from build123d import *

# Parameters (mm, degrees)
BOSS_EXTRUDE2_DEPTH = 5
BOSS_EXTRUDE3_DEPTH = 2
SKETCH4_W           = 3.2
SKETCH4_H           = 3.2
CUT_EXTRUDE1_DEPTH  = 2.5
SKETCH5_W           = 3.2
SKETCH5_H           = 3.2
CUT_EXTRUDE2_DEPTH  = 2.5
CUT_EXTRUDE4_REACH  = 34.123
CUT_EXTRUDE5_REACH  = 34.123
SKETCH8_W           = 2.5
SKETCH8_H           = 7
BOSS_EXTRUDE4_DEPTH = 5.96
SKETCH10_W          = 7
SKETCH10_H          = 2.49
BOSS_EXTRUDE5_DEPTH = 3
SKETCH11_W          = 7
SKETCH11_H          = 2.49
BOSS_EXTRUDE6_DEPTH = 5
SKETCH12_W          = 17
SKETCH12_H          = 2.5
BOSS_EXTRUDE7_DEPTH = 10
CUT_EXTRUDE7_REACH  = 41.734
SKETCH14_W          = 13
SKETCH14_H          = 8.75
SKETCH16_W          = 17
SKETCH16_H          = 1.25
BOSS_EXTRUDE8_DEPTH = 9.5
CUT_EXTRUDE8_REACH  = 34.394
SKETCH17_R          = 3.51
FILLET7_R           = 2
FILLET8_R           = 5
FILLET9_R           = 5
CHAMFER1_SIZE       = 2
CHAMFER2_SIZE       = 2
FILLET11_R          = 2
FILLET12_R          = 2
FILLET13_R          = 2
FILLET14_R          = 2
FILLET16_R          = 2


with BuildPart() as part:
    # Sketch2 → Boss-Extrude2 (new body)
    with BuildSketch(Plane.XY):
        Polygon((15.905331571, 19.450007488), (-15.905331571, 19.450007488), (-20.223253942, 15.132085117), (-21.991020895, 16.89985207), (-16.54629868, 22.344574285), (16.54629868, 22.344574285), (21.991020895, 16.89985207), (20.223253942, 15.132085117), align=None)
    extrude(amount=BOSS_EXTRUDE2_DEPTH)

    # Sketch2_2 → Boss-Extrude3 (add)
    with BuildSketch(Plane.XY):
        Polygon((15.905331571, 19.450007488), (-15.905331571, 19.450007488), (-20.223253942, 15.132085117), (-21.991020895, 16.89985207), (-16.54629868, 22.344574285), (16.54629868, 22.344574285), (21.991020895, 16.89985207), (20.223253942, 15.132085117), align=None)
    extrude(amount=-BOSS_EXTRUDE3_DEPTH)

    # Sketch4 → Cut-Extrude1 (cut)
    with BuildSketch(Plane(origin=(19.445436483, 19.445436483, 0), x_dir=(0.7071067811865479, -0.7071067811865471, 0), z_dir=(0.7071067811865471, 0.7071067811865479, 0))):
        with Locations((0, -1.5)):
            Rectangle(SKETCH4_W, SKETCH4_H)
    extrude(amount=-CUT_EXTRUDE1_DEPTH, mode=Mode.SUBTRACT)

    # Sketch5 → Cut-Extrude2 (cut)
    with BuildSketch(Plane(origin=(-19.445436483, 19.445436483, 0), x_dir=(0, 0, 1), z_dir=(-0.7071067811865477, 0.7071067811865475, 0))):
        with Locations((1.5, 0)):
            Rectangle(SKETCH5_W, SKETCH5_H)
    extrude(amount=-CUT_EXTRUDE2_DEPTH, mode=Mode.SUBTRACT)

    # Sketch6 → Cut-Extrude4 (cut, up to next)
    with BuildSketch(Plane.XY.offset(5), mode=Mode.PRIVATE) as cut_extrude4_sk1:
        Polygon((-20.011121908, 18.879751058), (-18.950461736, 19.940411229), (-17.182694783, 18.172644276), (-18.243354955, 17.111984105), align=None)
    cut_extrude4_tool1 = extrude(cut_extrude4_sk1.sketch, amount=-CUT_EXTRUDE4_REACH, mode=Mode.PRIVATE) & part.part
    add(cut_extrude4_tool1.solids().sort_by_distance((-18.596908, 18.526198, 5))[0], mode=Mode.SUBTRACT)

    # Sketch7 → Cut-Extrude5 (cut, up to next)
    with BuildSketch(Plane.XY.offset(5), mode=Mode.PRIVATE) as cut_extrude5_sk1:
        Polygon((17.182694783, 18.172644276), (18.950461736, 19.940411229), (20.011121908, 18.879751058), (18.243354955, 17.111984105), align=None)
    cut_extrude5_tool1 = extrude(cut_extrude5_sk1.sketch, amount=-CUT_EXTRUDE5_REACH, mode=Mode.PRIVATE) & part.part
    add(cut_extrude5_tool1.solids().sort_by_distance((18.596908, 18.526198, 5))[0], mode=Mode.SUBTRACT)

    # Sketch8 → Boss-Extrude4 (add)
    with BuildSketch(Plane(origin=(0, 19.450007488, 0), x_dir=(-1, 0, 0), z_dir=(0, -1, 0))):
        with Locations((11.1, -1.5)):
            Rectangle(SKETCH8_W, SKETCH8_H)
        with Locations((-11.1, -1.5)):
            Rectangle(SKETCH8_W, SKETCH8_H)
    extrude(amount=BOSS_EXTRUDE4_DEPTH)

    # Sketch10 → Boss-Extrude5 (add)
    with BuildSketch(Plane.ZY.offset(-9.85)):
        with Locations((1.5, 14.735007488)):
            Rectangle(SKETCH10_W, SKETCH10_H)
    extrude(amount=BOSS_EXTRUDE5_DEPTH)

    # Sketch11 → Boss-Extrude6 (add)
    with BuildSketch(Plane(origin=(-9.85, 0, 0), x_dir=(0, 0, -1), z_dir=(1, 0, 0))):
        with Locations((-1.5, 14.735007488)):
            Rectangle(SKETCH11_W, SKETCH11_H)
    extrude(amount=BOSS_EXTRUDE6_DEPTH)

    # Sketch12 → Boss-Extrude7 (add)
    with BuildSketch(Plane(origin=(0, 22.344574285, 0), x_dir=(1, 0, 0), z_dir=(0, 1, 0))):
        with Locations((0, -3.75)):
            Rectangle(SKETCH12_W, SKETCH12_H)
    extrude(amount=BOSS_EXTRUDE7_DEPTH)

    # Sketch14 → Cut-Extrude7 (cut, up to next)
    with BuildSketch(Plane.XY.offset(5), mode=Mode.PRIVATE) as cut_extrude7_sk1:
        with Locations((0, 26.719574285)):
            Rectangle(SKETCH14_W, SKETCH14_H)
    cut_extrude7_tool1 = extrude(cut_extrude7_sk1.sketch, amount=-CUT_EXTRUDE7_REACH, mode=Mode.PRIVATE) & part.part
    add(cut_extrude7_tool1.solids().sort_by_distance((0, 26.719574, 5))[0], mode=Mode.SUBTRACT)

    # Sketch16 → Boss-Extrude8 (add)
    with BuildSketch(Plane.XY.offset(5)):
        with Locations((0, 31.719574285)):
            Rectangle(SKETCH16_W, SKETCH16_H)
    extrude(amount=BOSS_EXTRUDE8_DEPTH)

    # Sketch17 → Cut-Extrude8 (cut, up to next)
    with BuildSketch(Plane(origin=(0, 32.344574285, 0), x_dir=(1, 0, 0), z_dir=(0, 1, 0)), mode=Mode.PRIVATE) as cut_extrude8_sk1:
        with Locations(Location((0, -9, 0), (0, 0, 270))):
            Circle(SKETCH17_R)
    cut_extrude8_tool1 = extrude(cut_extrude8_sk1.sketch, amount=-CUT_EXTRUDE8_REACH, mode=Mode.PRIVATE) & part.part
    add(cut_extrude8_tool1.solids().sort_by_distance((0, 32.344574, 9))[0], mode=Mode.SUBTRACT)

    # Fillet7
    fillet7_edges = [part.edges().sort_by_distance(p)[0] for p in [
        (7.5, 31.094574285, 5),
    ]]
    fillet(fillet7_edges, radius=FILLET7_R)

    # Fillet8
    fillet8_edges = [part.edges().sort_by_distance(p)[0] for p in [
        (8.5, 31.719574285, 14.5),
    ]]
    fillet(fillet8_edges, radius=FILLET8_R)

    # Fillet9
    fillet9_edges = [part.edges().sort_by_distance(p)[0] for p in [
        (-8.5, 31.719574285, 14.5),
    ]]
    fillet(fillet9_edges, radius=FILLET9_R)

    # Chamfer1
    chamfer1_edges = [part.edges().sort_by_distance(p)[0] for p in [
        (-12.35, 13.490007488, 1.5),
    ]]
    chamfer(chamfer1_edges, length=CHAMFER1_SIZE)

    # Chamfer2
    chamfer2_edges = [part.edges().sort_by_distance(p)[0] for p in [
        (12.35, 13.490007488, 1.5),
    ]]
    chamfer(chamfer2_edges, length=CHAMFER2_SIZE)

    # Fillet11
    fillet11_edges = [part.edges().sort_by_distance(p)[0] for p in [
        (-8.5, 22.344574285, 3.75),
    ]]
    fillet(fillet11_edges, radius=FILLET11_R)

    # Fillet12
    fillet12_edges = [part.edges().sort_by_distance(p)[0] for p in [
        (8.5, 22.344574285, 3.75),
    ]]
    fillet(fillet12_edges, radius=FILLET12_R)

    # Fillet13
    fillet13_edges = [part.edges().sort_by_distance(p)[0] for p in [
        (8.5, 22.344574285, 2.5),
    ]]
    fillet(fillet13_edges, radius=FILLET13_R)

    # Fillet14
    fillet14_edges = [part.edges().sort_by_distance(p)[0] for p in [
        (-8.5, 22.344574285, 2.5),
    ]]
    fillet(fillet14_edges, radius=FILLET14_R)

    # Fillet16
    fillet16_edges = [part.edges().sort_by_distance(p)[0] for p in [
        (-7.5, 31.094574285, 5),
    ]]
    fillet(fillet16_edges, radius=FILLET16_R)


solid = part.part
The listing builds one solid part. Answer for the finished solid, in the listing's coordinates (mm). A direction names the side the tool comes from. Give positions to 0.01 mm unless a question says otherwise; leave off trailing zeros. Write each loop counter-clockwise with the first axis right and the second up, starting at its lowest first coordinate (ties: lowest second). Pieces come first, ordered by that corner, then holes. Notation, with made-up numbers: (-31, -9.75) -> (13, -9.75) arc R32 cw to (13, 26.25) -> close; hole circle Ø1 at (17.25, 21). An arc over 180 degrees is marked (long way). One line per question, with ' | ' between items. Start each with the question number.
1. Section D-D (x = 7.5) is taken. Determine the outline of the cut face in (y, z).
2. Given pin 1 Ø3.5 at (x, z) = (2.5, 7) entering from -Y; pin 2 Ø4.5 at (y, z) = (17, 1.5) entering from +X; pin 3 Ø5 at (y, z) = (20, 2) entering from +X; pin 4 Ø1.5 at (x, z) = (14.5, 3) entering from +Y, each flat-ended and moving along its own axis, determine where each tip first touches the part or whether it passes through.
3. Section B-B (x = 0) is taken. Determine the outline of the cut face in (y, z), plus the area to 3 significant figures.
4. Section C-C (y = 30.5) is taken. Determine the outline of the cut face in (x, z), plus the area to 3 significant figures.
5. Section A-A (z = 9) is taken. Determine the outline of the cut face in (x, y), plus the area to 3 significant figures.
6. For a pull along Y with two mould halves and no side action, classify faces 1 (the flat face through (8, 15.98, 1)), 2 (the flat face through (17.443, 19.705, 1.522)), 3 (the flat face through (19.4, 17.7, 3.1)) as pulls with the +Y half, pulls with the -Y half, needs draft (parallel to the pull), parting line crosses it, or undercut.
7. Find the intervals of material crossed by probe 1 along X at (y, z) = (31.6, 9); probe 2 along Y at (x, z) = (-5, 12); probe 3 along Y at (x, z) = (-7, -1), in increasing order.
8. For faces 4 (the flat face through (0, 32, 2.5)), 5 (the flat face through (-14, 19.45, 2)), 6 (the flat face through (-18.08, 19.07, 4.06)), 7 (the flat face through (0, 21, 5)), 8 (the flat face through (-19.705, 17.443, 1.478)), determine the directions among +Z, -Z, +X, -X, +Y, -Y from which every point of the face is accessible in a straight line to the end or side of a thin tool.
Response values:
1) outline: (13.49, -2) -> (15.98, -2) -> (15.98, 5) -> (13.49, 5) -> close; (19.45, -2) -> (22.34, -2) -> (22.34, 0.5) arc R2 cw to (24.34, 2.5) -> (32.34, 2.5) -> (32.34, 12.5) -> (31.09, 12.5) -> (31.09, 7) arc R2 cw to (29.09, 5) -> (19.45, 5) -> close
2) pin 1: y = 31.09 | pin 2: x = 21.99 | pin 3: x = 21.39 | pin 4: y = 22.34
3) outline: (19.45, -2) -> (22.34, -2) -> (22.34, 5) -> (19.45, 5) -> close; (31.09, 2.5) -> (32.34, 2.5) -> (32.34, 5.49) -> (31.09, 5.49) -> close; (31.09, 12.51) -> (32.34, 12.51) -> (32.34, 14.5) -> (31.09, 14.5) -> close | area: 26.5 mm2
4) outline: (-8.5, 2.5) -> (-6.5, 2.5) -> (-6.5, 5.58) -> (-8.5, 5.58) -> close; (6.5, 2.5) -> (8.5, 2.5) -> (8.5, 5.58) -> (6.5, 5.58) -> close | area: 12.3 mm2
5) outline: (-8.5, 31.09) -> (-3.51, 31.09) -> (-3.51, 32.34) -> (-8.5, 32.34) -> close; (3.51, 31.09) -> (8.5, 31.09) -> (8.5, 32.34) -> (3.51, 32.34) -> close | area: 12.5 mm2
6) face 1: undercut | face 2: pulls with the -Y half | face 3: needs draft
7) probe 1: -8.5 to -3.51, 3.51 to 8.5 | probe 2: 31.09 to 32.34 | probe 3: 13.49 to 15.98, 19.45 to 22.34
8) face 4: -Z, +X, -X, +Y | face 5: +Z, -Z, -Y | face 6: +Z | face 7: +Z, +X, -X, -Y | face 8: +Y
